```python
from build123d import *

# Parameters (mm, degrees)
SKETCH1_R           = 63.5
BOSS_EXTRUDE1_DEPTH = 6.35
SKETCH2_R           = 4.445
BOSS_EXTRUDE2_DEPTH = 8.89
SKETCH1_3_R         = 4.445
BOSS_EXTRUDE3_DEPTH = 6.35
SKETCH3_R           = 7.665246074
BOSS_EXTRUDE4_DEPTH = 2.54


with BuildPart() as part:
    # Sketch1 → Boss-Extrude1 (new body)
    with BuildSketch(Plane.XY):
        Circle(SKETCH1_R)
    extrude(amount=BOSS_EXTRUDE1_DEPTH)

    # Sketch2 → Boss-Extrude2 (add)
    with BuildSketch(Plane.XY.offset(6.35)):
        with Locations((45.72, 0)):
            Circle(SKETCH2_R)
    extrude(amount=BOSS_EXTRUDE2_DEPTH)

    # Sketch1<3> → Boss-Extrude3 (add)
    with BuildSketch(Plane.XY):
        Circle(SKETCH1_3_R)
    extrude(amount=-BOSS_EXTRUDE3_DEPTH)

    # Sketch3 → Boss-Extrude4 (add)
    with BuildSketch(Plane(origin=(0, 0, -6.35), x_dir=(-1, 0, 0), z_dir=(0, 0, -1))):
        Circle(SKETCH3_R)
    extrude(amount=BOSS_EXTRUDE4_DEPTH)


solid = part.part
```
Geometry check sheet. Reference: the model listing, model coordinates, mm. A direction names the side the tool comes from. Coordinates: 2 decimals unless noted, no trailing zeros. Order: outer loops, then holes, each group sorted by start corner. A loop starts at its lowest first (then second) coordinate and runs counter-clockwise, first axis right, second up. Notation, with made-up numbers: M 40,76.5 L 87,76.5 A31 cw 87,115.5 Z; hole C 32,87 d4. An arc over 180 degrees is marked long. One line per question, with ' | ' between items. Start each with the question number.
Item 1: Material ranges on L1, parallel to Z at x = -39, y = -2.5; L2, parallel to Y at x = 3, z = 4.75; L3, parallel to Y at x = 24, z = 5, recorded low to high. Write a range as [from, to].
Item 2: Set-up check for faces 1 (the flat face through (46, 0, 15.24)), 2 (the cylindrical face through (41.28, 0.2, 10.73)), 3 (the cylindrical face through (1.662, -7.483, -7.602)), 4 (the flat face through (-3.3, -3.3, -6.35)): record each of +Z, -Z, +X, -X, +Y, -Y from which the full face is reachable in a straight line by a thin tool's end or side.
Item 3: Cross-section at C-C on z = -3. Enter the section's corners in (x, y) (3 decimals).
Item 4: Cross-section at D-D on x = 45.72. Enter the section's corners in (y, z) (3 decimals), then the cut area to 3 significant figures.
Item 5: Gauge pin test, flat ends, axial feed: pin 1 (10 mm diameter, centred on x = -26, z = 0, fed in from -Y); pin 2 (1 mm diameter, centred on y = 11, z = 5.5, fed in from +X); pin 3 (1.5 mm diameter, centred on x = -19.5, y = 5, fed in from +Z). Record the tip position at first contact, or that the pin passes through.
Item 6: Cross-section at B-B on x = 0. Enter the section's corners in (y, z) (3 decimals).
Item 7: Cross-section at A-A on y = 0. Enter the section's corners in (x, z) (3 decimals).
Findings:
1) L1: z = [0, 6.35] | L2: y = [-63.43, 63.43] | L3: y = [-58.79, 58.79]
2) face 1: +Z, +X, -X, +Y, -Y | face 2: +Z | face 3: -Z | face 4: none
3) outline: C 0,0 d8.89
4) outline: M -44.067,0 L 44.067,0 L 44.067,6.35 L 4.445,6.35 L 4.445,15.24 L -4.445,15.24 L -4.445,6.35 L -44.067,6.35 Z | area: 639 mm²
5) pin 1: stops at y = -59.93 | pin 2: stops at x = 62.63 | pin 3: stops at z = 6.35
6) outline: M -63.5,0 L -4.445,0 L -4.445,-6.35 L -7.665,-6.35 L -7.665,-8.89 L 7.665,-8.89 L 7.665,-6.35 L 4.445,-6.35 L 4.445,0 L 63.5,0 L 63.5,6.35 L -63.5,6.35 Z
7) outline: M -63.5,0 L -4.445,0 L -4.445,-6.35 L -7.665,-6.35 L -7.665,-8.89 L 7.665,-8.89 L 7.665,-6.35 L 4.445,-6.35 L 4.445,0 L 63.5,0 L 63.5,6.35 L 50.165,6.35 L 50.165,15.24 L 41.275,15.24 L 41.275,6.35 L -63.5,6.35 Z
